```python
from build123d import *

# Parameters (mm, degrees)
EXTRUDE_1_DEPTH     = 105
SKETCH_3_W          = 107.6
SKETCH_3_H          = 1.2
EXTRUDE_3_DEPTH     = 36
SKETCH_4_R          = 3
SKETCH_4_W          = 70
SKETCH_4_H          = 1
EXTRUDE_4_DEPTH     = 5
CUT_EXTRUDE_1_REACH = 129.213
CUT_EXTRUDE_START   = -1
SKETCH_5_R          = 1.5
SKETCH_6_R          = 1.75
SKETCH_6_W          = 6
SKETCH_6_H          = 81
CUT_EXTRUDE_2_DEPTH = 10
EXTRUDE_8_DEPTH     = 82
EXTRUDE_9_DEPTH     = 1
EXTRUDE_10_DEPTH    = 1
CUT_EXTRUDE_3_REACH = 128.836
SKETCH_11_W         = 18
SKETCH_11_H         = 15
CUT_EXTRUDE_4_REACH = 129.82
SKETCH_12_R         = 1.5
SKETCH_12_W         = 30
SKETCH_12_H         = 15
EXTRUDE_11_DEPTH    = 50
SKETCH_14_W         = 20
SKETCH_14_H         = 14.8
EXTRUDE_12_DEPTH    = 2
SKETCH_15_W         = 6
SKETCH_15_H         = 10
SKETCH_15_W_2       = 3
SKETCH_15_H_2       = 6
EXTRUDE_13_DEPTH    = 2
CUT_EXTRUDE_5_REACH = 139.208
SKETCH_16_W         = 6
SKETCH_16_H         = 4


with BuildPart() as part:
    # 草图1 → 凸台-拉伸1 (new body)
    with BuildSketch(Plane.XY):
        Polygon((-54.8, 0), (54.8, 0), (54.8, 35.8), (62.8, 35.8), (62.8, 37), (53.8, 37), (53.8, 1), (17.4, 1), (17.4, 16), (16.2, 16), (16.2, 1), (-53.8, 1), (-53.8, 37), (-62.8, 37), (-62.8, 35.8), (-54.8, 35.8), align=None)
    extrude(amount=EXTRUDE_1_DEPTH)

    # 草图3 → 凸台-拉伸3 (add)
    with BuildSketch(Plane(origin=(0, 1, 0), x_dir=(1, 0, 0), z_dir=(0, 1, 0))):
        with Locations((0, -0.6)):
            Rectangle(SKETCH_3_W, SKETCH_3_H)
        with Locations((0, -104.4)):
            Rectangle(SKETCH_3_W, SKETCH_3_H)
    extrude(amount=EXTRUDE_3_DEPTH)

    # 草图4 → 凸台-拉伸4 (add)
    with BuildSketch(Plane(origin=(0, 1, 0), x_dir=(1, 0, 0), z_dir=(0, 1, 0))):
        with Locations((20, -89)):
            Circle(SKETCH_4_R)
        with Locations((-20, -89)):
            Circle(SKETCH_4_R)
        with Locations((-18.8, -21.7)):
            Rectangle(SKETCH_4_W, SKETCH_4_H)
        with Locations((-18.8, -42.7)):
            Rectangle(SKETCH_4_W, SKETCH_4_H)
        with Locations((-18.8, -62.3)):
            Rectangle(SKETCH_4_W, SKETCH_4_H)
        with Locations((-18.8, -83.3)):
            Rectangle(SKETCH_4_W, SKETCH_4_H)
    extrude(amount=EXTRUDE_4_DEPTH)

    # 草图5 → 切除-拉伸1 (cut, up to next)
    with BuildSketch(Plane(origin=(0, 6, 0), x_dir=(1, 0, 0), z_dir=(0, 1, 0)).offset(CUT_EXTRUDE_START), mode=Mode.PRIVATE) as cut_extrude_1_sk1:
        with Locations(Location((20, -89, 0), (0, 0, 180))):
            Circle(SKETCH_5_R)
    cut_extrude_1_tool1 = extrude(cut_extrude_1_sk1.sketch, amount=-CUT_EXTRUDE_1_REACH, mode=Mode.PRIVATE) & part.part
    # 草图5 → 切除-拉伸1 (cut, up to next)
    with BuildSketch(Plane(origin=(0, 6, 0), x_dir=(1, 0, 0), z_dir=(0, 1, 0)).offset(CUT_EXTRUDE_START), mode=Mode.PRIVATE) as cut_extrude_1_sk2:
        with Locations(Location((-20, -89, 0), (0, 0, 180))):
            Circle(SKETCH_5_R)
    cut_extrude_1_tool2 = extrude(cut_extrude_1_sk2.sketch, amount=-CUT_EXTRUDE_1_REACH, mode=Mode.PRIVATE) & part.part
    add(cut_extrude_1_tool1.solids().sort_by_distance((20, 5, 89))[0], mode=Mode.SUBTRACT)
    add(cut_extrude_1_tool2.solids().sort_by_distance((-20, 5, 89))[0], mode=Mode.SUBTRACT)

    # 草图6 → 切除-拉伸2 (cut)
    with BuildSketch(Plane(origin=(0, 37, 0), x_dir=(1, 0, 0), z_dir=(0, 1, 0))):
        with Locations(Location((58.8, -5, 0), (0, 0, 270))):
            Circle(SKETCH_6_R)
        with Locations(Location((58.8, -99, 0), (0, 0, 270))):
            Circle(SKETCH_6_R)
        with Locations(Location((-58.8, -99, 0), (0, 0, 180))):
            Circle(SKETCH_6_R)
        with Locations(Location((-58.8, -5, 0), (0, 0, 180))):
            Circle(SKETCH_6_R)
        with Locations((-56.8, -52.5)):
            Rectangle(SKETCH_6_W, SKETCH_6_H)
        with Locations((56.8, -52.5)):
            Rectangle(SKETCH_6_W, SKETCH_6_H)
    extrude(amount=-CUT_EXTRUDE_2_DEPTH, mode=Mode.SUBTRACT)

    # 草图7 → 凸台-拉伸8 (add)
    with BuildSketch(Plane.XY.offset(12)):
        Polygon((60.950143721, 35.8), (54.8, 24.975747051), (54.8, 27), (59.8, 35.8), align=None)
        Polygon((-54.8, 24.975747051), (-54.8, 27), (-59.8, 35.8), (-60.950143721, 35.8), align=None)
    extrude(amount=EXTRUDE_8_DEPTH)

    # 草图8 → 凸台-拉伸9 (add)
    with BuildSketch(Plane(origin=(0, 0, 12), x_dir=(-1, 0, 0), z_dir=(0, 0, -1))):
        Polygon((-54.8, 35.8), (-60.950143721, 35.8), (-54.8, 24.975747051), align=None)
        Polygon((54.8, 24.975747051), (54.8, 35.8), (60.950143721, 35.8), align=None)
    extrude(amount=EXTRUDE_9_DEPTH)

    # 草图10 → 凸台-拉伸10 (add)
    with BuildSketch(Plane.XY.offset(94)):
        Polygon((-60.950143721, 35.8), (-54.8, 35.8), (-54.8, 24.975747051), align=None)
        Polygon((54.8, 24.975747051), (60.950143721, 35.8), (54.8, 35.8), align=None)
    extrude(amount=EXTRUDE_10_DEPTH)

    # 草图11 → 切除-拉伸3 (cut, up to next)
    with BuildSketch(Plane.XY.offset(1.2), mode=Mode.PRIVATE) as cut_extrude_3_sk1:
        with Locations((0, 29.5)):
            Rectangle(SKETCH_11_W, SKETCH_11_H)
    cut_extrude_3_tool1 = extrude(cut_extrude_3_sk1.sketch, amount=-CUT_EXTRUDE_3_REACH, mode=Mode.PRIVATE) & part.part
    add(cut_extrude_3_tool1.solids().sort_by_distance((0, 29.5, 1.2))[0], mode=Mode.SUBTRACT)

    # 草图12 → 切除-拉伸4 (cut, up to next)
    with BuildSketch(Plane.XY.offset(105), mode=Mode.PRIVATE) as cut_extrude_4_sk1:
        with Locations((50, 5)):
            Circle(SKETCH_12_R)
    cut_extrude_4_tool1 = extrude(cut_extrude_4_sk1.sketch, amount=-CUT_EXTRUDE_4_REACH, mode=Mode.PRIVATE) & part.part
    # 草图12 → 切除-拉伸4 (cut, up to next)
    with BuildSketch(Plane.XY.offset(105), mode=Mode.PRIVATE) as cut_extrude_4_sk2:
        with Locations((50, 33)):
            Circle(SKETCH_12_R)
    cut_extrude_4_tool2 = extrude(cut_extrude_4_sk2.sketch, amount=-CUT_EXTRUDE_4_REACH, mode=Mode.PRIVATE) & part.part
    # 草图12 → 切除-拉伸4 (cut, up to next)
    with BuildSketch(Plane.XY.offset(105), mode=Mode.PRIVATE) as cut_extrude_4_sk3:
        with Locations((-50, 33)):
            Circle(SKETCH_12_R)
    cut_extrude_4_tool3 = extrude(cut_extrude_4_sk3.sketch, amount=-CUT_EXTRUDE_4_REACH, mode=Mode.PRIVATE) & part.part
    # 草图12 → 切除-拉伸4 (cut, up to next)
    with BuildSketch(Plane.XY.offset(105), mode=Mode.PRIVATE) as cut_extrude_4_sk4:
        with Locations((-50, 5)):
            Circle(SKETCH_12_R)
    cut_extrude_4_tool4 = extrude(cut_extrude_4_sk4.sketch, amount=-CUT_EXTRUDE_4_REACH, mode=Mode.PRIVATE) & part.part
    # 草图12 → 切除-拉伸4 (cut, up to next)
    with BuildSketch(Plane.XY.offset(105), mode=Mode.PRIVATE) as cut_extrude_4_sk5:
        with Locations((15, 29.5)):
            Rectangle(SKETCH_12_W, SKETCH_12_H)
    cut_extrude_4_tool5 = extrude(cut_extrude_4_sk5.sketch, amount=-CUT_EXTRUDE_4_REACH, mode=Mode.PRIVATE) & part.part
    add(cut_extrude_4_tool1.solids().sort_by_distance((50, 5, 105))[0], mode=Mode.SUBTRACT)
    add(cut_extrude_4_tool2.solids().sort_by_distance((50, 33, 105))[0], mode=Mode.SUBTRACT)
    add(cut_extrude_4_tool3.solids().sort_by_distance((-50, 33, 105))[0], mode=Mode.SUBTRACT)
    add(cut_extrude_4_tool4.solids().sort_by_distance((-50, 5, 105))[0], mode=Mode.SUBTRACT)
    add(cut_extrude_4_tool5.solids().sort_by_distance((15, 29.5, 105))[0], mode=Mode.SUBTRACT)

    # 草图13 → 凸台-拉伸11 (add)
    with BuildSketch(Plane(origin=(0, 0, 0), x_dir=(-1, 0, 0), z_dir=(0, 0, -1))):
        Polygon((9, 35.8), (9, 22), (-9, 22), (-9, 35.8), (-10, 35.8), (-10, 21), (10, 21), (10, 35.8), align=None)
    extrude(amount=EXTRUDE_11_DEPTH)

    # 草图14 → 凸台-拉伸12 (add)
    with BuildSketch(Plane(origin=(0, 0, -50), x_dir=(-1, 0, 0), z_dir=(0, 0, -1))):
        with Locations((0, 28.4)):
            Rectangle(SKETCH_14_W, SKETCH_14_H)
    extrude(amount=EXTRUDE_12_DEPTH)

    # 草图15 → 凸台-拉伸13 (add)
    # profile 1 of 2: a face of its own
    with BuildSketch(Plane(origin=(0, 27, 0), x_dir=(1, 0, 0), z_dir=(0, 1, 0))):
        with Locations((-51.8, -27.5)):
            Rectangle(SKETCH_15_W, SKETCH_15_H)
        with Locations((-52.3, -27.5)):
            Rectangle(SKETCH_15_W_2, SKETCH_15_H_2, mode=Mode.SUBTRACT)
    # profile 2 of 2: a face of its own
    with BuildSketch(Plane(origin=(0, 27, 0), x_dir=(1, 0, 0), z_dir=(0, 1, 0))):
        with Locations((-51.8, -77.5)):
            Rectangle(SKETCH_15_W, SKETCH_15_H)
        with Locations((-52.3, -77.5)):
            Rectangle(SKETCH_15_W_2, SKETCH_15_H_2, mode=Mode.SUBTRACT)
    extrude(amount=-EXTRUDE_13_DEPTH)

    # 草图16 → 切除-拉伸5 (cut, up to next)
    with BuildSketch(Plane(origin=(17.4, 0, 0), x_dir=(0, 0, -1), z_dir=(1, 0, 0)), mode=Mode.PRIVATE) as cut_extrude_5_sk1:
        with Locations((-76, 12)):
            Rectangle(SKETCH_16_W, SKETCH_16_H)
    cut_extrude_5_tool1 = extrude(cut_extrude_5_sk1.sketch, amount=-CUT_EXTRUDE_5_REACH, mode=Mode.PRIVATE) & part.part
    # 草图16 → 切除-拉伸5 (cut, up to next)
    with BuildSketch(Plane(origin=(17.4, 0, 0), x_dir=(0, 0, -1), z_dir=(1, 0, 0)), mode=Mode.PRIVATE) as cut_extrude_5_sk2:
        with Locations((-30, 12)):
            Rectangle(SKETCH_16_W, SKETCH_16_H)
    cut_extrude_5_tool2 = extrude(cut_extrude_5_sk2.sketch, amount=-CUT_EXTRUDE_5_REACH, mode=Mode.PRIVATE) & part.part
    add(cut_extrude_5_tool1.solids().sort_by_distance((17.4, 12, 76))[0], mode=Mode.SUBTRACT)
    add(cut_extrude_5_tool2.solids().sort_by_distance((17.4, 12, 30))[0], mode=Mode.SUBTRACT)


solid = part.part
```
Build history of the part. All positions in model axes, mm. A direction names the side the tool comes from. Give positions to 0.01 mm unless a question says otherwise; leave off trailing zeros. Order: outer loops, then holes, each group sorted by start corner. A loop starts at its lowest first (then second) coordinate and runs counter-clockwise, first axis right, second up. Notation, with made-up numbers: M 27.5,52.5 L 66.5,52.5 A13 ccw 66.5,75.5 Z; hole C 82.5,-14.75 d2. An arc over 180 degrees is marked long. Return JSON: item names as keys, results as strings.
Q1. Band-saw the part on C-C (z = -9.5). Give the cut face in (x, y), then the cut area to 3 significant figures.
Answer list:
{"outline": "M -10,21 L 10,21 L 10,35.8 L 9,35.8 L 9,22 L -9,22 L -9,35.8 L -10,35.8 Z", "area": "47.6 mm^2"}
Q2. Wall check: probe 1 along Y at (x, z) = (50, 104); probe 2 along X at (y, z) = (8.5, 34); probe 3 along X at (y, z) = (3, 89). Give the ranges that are in metal, low to high. Write a range as from..to.
Answer list:
{"probe 1": "y = 0..3.5, 6.5..31.5, 34.5..37", "probe 2": "x = -54.8..-53.8, 16.2..17.4, 53.8..54.8", "probe 3": "x = -54.8..-53.8, -23..-21.5, -18.5..-17, 16.2..18.5, 21.5..23, 53.8..54.8"}
Q3. Flat gauge pins, fed straight in: pin 1 (1.6 mm diameter, centred on x = -51.5, y = 26, fed in from -Z); pin 2 (5 mm diameter, centred on x = -3.5, z = -30, fed in from -Y); pin 3 (4.5 mm diameter, centred on y = 6, z = 33, fed in from -X). Where does each tip first touch, or does it go through?
Answer list:
{"pin 1": "stops at z = 0", "pin 2": "stops at y = 21", "pin 3": "stops at x = -54.8"}
Q4. Band-saw the part on B-B (x = -38). Give the cut face in (y, z), then the cut area to 3 significant figures.
Answer list:
{"outline": "M 0,0 L 37,0 L 37,1.2 L 1,1.2 L 1,21.2 L 6,21.2 L 6,22.2 L 1,22.2 L 1,42.2 L 6,42.2 L 6,43.2 L 1,43.2 L 1,61.8 L 6,61.8 L 6,62.8 L 1,62.8 L 1,82.8 L 6,82.8 L 6,83.8 L 1,83.8 L 1,103.8 L 37,103.8 L 37,105 L 0,105 Z", "area": "211 mm^2"}
Q5. Two-plate mould, pull along X, no slides. Class faces 1 (the face through (-57.83, 30.31, 52.41)), 2 (the face through (57.83, 30.31, 52.41)), 3 (the face through (-20, 6, 89)): pulls with the +X half, pulls with the -X half, needs draft (parallel to the pull), parting line crosses it, or undercut.
Answer list:
{"face 1": "pulls with the -X half", "face 2": "pulls with the +X half", "face 3": "undercut"}
Q6. 3-axis set-ups, long thin cutter, end or side, ignore diameter. For faces 4 (the face through (-50, 25, 77)), 5 (the face through (-61.2, 35.8, 52.3)), 6 (the face through (-19, 3, 22.2)), 7 (the face through (10, 28, -26)): which of +Z, -Z, +X, -X, +Y, -Y reach the whole face in a straight line?
Answer list:
{"face 4": "none", "face 5": "-X, -Y", "face 6": "+Y", "face 7": "-Z, +X, +Y, -Y"}
Q7. Band-saw the part on A-A (z = 99). Give the cut face in (x, y), then the cut area to 3 significant figures.
Answer list:
{"outline": "M -62.8,35.8 L -60.55,35.8 L -60.55,37 L -62.8,37 Z; M -57.05,35.8 L -54.8,35.8 L -54.8,0 L 54.8,0 L 54.8,35.8 L 57.05,35.8 L 57.05,37 L 53.8,37 L 53.8,1 L 17.4,1 L 17.4,16 L 16.2,16 L 16.2,1 L -53.8,1 L -53.8,37 L -57.05,37 Z; M 60.55,35.8 L 62.8,35.8 L 62.8,37 L 60.55,37 Z", "area": "210 mm^2"}
